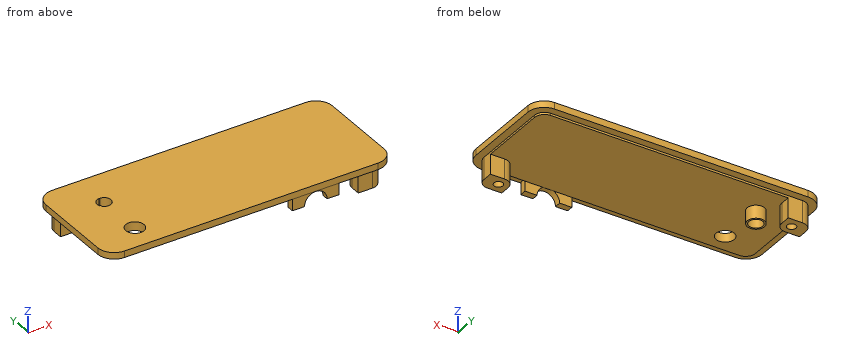
```python
from build123d import *

# Parameters (mm, degrees)
PAD002_DEPTH  = 1.5
PAD003_DEPTH  = 0.5
SKETCH005_R   = 1.025
PAD004_DEPTH  = 4.6
SKETCH006_R   = 2.1
POCKET_DEPTH  = 2
SKETCH008_R   = 2
SKETCH008_R_2 = 1.6
PAD005_DEPTH  = 3
PAD014_DEPTH  = 1.5


with BuildPart() as part:
    # Sketch003 → Pad002 (new body)
    with BuildSketch(Plane.XY.offset(6)):
        with BuildLine():
            Line((-29.25, 13), (29.25, 13))
            ThreePointArc((33, 9.25), (31.9016504294, 11.9016504294), (29.25, 13))
            Line((33, 9.25), (33, -9.25))
            ThreePointArc((29.25, -13), (31.9016504295, -11.9016504294), (33, -9.25))
            Line((29.25, -13), (-29.25, -13))
            ThreePointArc((-33, -9.25), (-31.9016504294, -11.9016504295), (-29.25, -13))
            Line((-33, -9.25), (-33, 9.25))
            ThreePointArc((-29.25, 13), (-31.9016504294, 11.9016504294), (-33, 9.25))
        make_face()
    extrude(amount=PAD002_DEPTH)

    # Sketch004 → Pad003 (new body)
    with BuildSketch(Plane(origin=(0, 0, 6), x_dir=(1, 0, 0), z_dir=(0, 0, -1))):
        with BuildLine():
            Line((-29.05, 11.3), (29.05, 11.3))
            ThreePointArc((31.3, 9.05), (30.6409902577, 10.6409902577), (29.05, 11.3))
            Line((31.3, 9.05), (31.3, -9.05))
            ThreePointArc((29.05, -11.3), (30.6409902577, -10.6409902577), (31.3, -9.05))
            Line((29.05, -11.3), (-29.05, -11.3))
            ThreePointArc((-31.3, -9.05), (-30.6409902577, -10.6409902577), (-29.05, -11.3))
            Line((-31.3, -9.05), (-31.3, 9.05))
            ThreePointArc((-29.05, 11.3), (-30.6409902577, 10.6409902577), (-31.3, 9.05))
        make_face()
    extrude(amount=PAD003_DEPTH)

    # Sketch005 → Pad004 (new body)
    with BuildSketch(Plane(origin=(0, 0, 5.5), x_dir=(1, 0, 0), z_dir=(0, 0, -1))):
        with BuildLine():
            Line((-25.75, -9), (-25.75, -11.3))
            Line((-25.75, -11.3), (-29.05, -11.3))
            ThreePointArc((-31.3, -9.05), (-30.6409902577, -10.6409902577), (-29.05, -11.3))
            Line((-31.3, -6.75), (-31.3, -9.05))
            Line((-27.9999999923, -6.75), (-31.3, -6.75))
            ThreePointArc((-25.75, -9.0000000077), (-26.4090097369, -7.4090097478), (-27.9999999923, -6.75))
        make_face()
        with Locations((-28, -9)):
            Circle(SKETCH005_R, mode=Mode.SUBTRACT)
        with BuildLine():
            ThreePointArc((25.75, 9), (26.4090097423, 7.4090097423), (28, 6.75))
            Line((28, 6.75), (31.3, 6.75))
            Line((31.3, 9.05), (31.3, 6.75))
            ThreePointArc((31.3, 9.05), (30.6409902577, 10.6409902577), (29.05, 11.3))
            Line((29.05, 11.3), (25.75, 11.3))
            Line((25.75, 11.3), (25.75, 9))
        make_face()
        with Locations((28, 9)):
            Circle(SKETCH005_R, mode=Mode.SUBTRACT)
    extrude(amount=PAD004_DEPTH)

    # Sketch006 → Pocket (cut)
    with BuildSketch(Plane.XY.offset(7.5)):
        with Locations((-23, -7)):
            Circle(SKETCH006_R)
        with BuildLine():
            ThreePointArc((-24.3288922086, 3.1089076939), (-23.0026761128, 2.400002238), (-21.6740960519, 3.1044673539))
            ThreePointArc((-21.5638430432, 3.2946963807), (-21.7108688116, 3.2528448762), (-21.6740960519, 3.1044673539))
            ThreePointArc((-21.5638430432, 3.2946963807), (-21.6130238799, 4.7976824194), (-22.8873953748, 5.5960326433))
            ThreePointArc((-23.1072650483, 5.5964003913), (-22.9975078699, 5.4899979159), (-22.8873953748, 5.5960326433))
            ThreePointArc((-23.1072650483, 5.5964003913), (-24.3843000035, 4.8023175806), (-24.4385082583, 3.2995044678))
            ThreePointArc((-24.3288922086, 3.1089076939), (-24.2916233116, 3.2571613762), (-24.4385082583, 3.2995044678))
        make_face()
    extrude(amount=-POCKET_DEPTH, mode=Mode.SUBTRACT)

    # Sketch008 → Pad005 (new body)
    with BuildSketch(Plane(origin=(0, 0, 5.5), x_dir=(1, 0, 0), z_dir=(0, 0, -1))):
        with Locations((-23, -4)):
            Circle(SKETCH008_R)
        with Locations((-23, -4)):
            Circle(SKETCH008_R_2, mode=Mode.SUBTRACT)
    extrude(amount=PAD005_DEPTH)

    # Sketch023 → Pad014 (new body)
    with BuildSketch(Plane(origin=(0, -11.3, 6), x_dir=(1, 0, 0), z_dir=(0, -1, 0))):
        with BuildLine():
            Line((9.6, 0), (20.4, 0))
            Line((20.4, 0), (20.4, -2.8))
            Line((20.4, -2.8), (17.6, -2.8))
            ThreePointArc((17.6, -2.8), (15, -0.2), (12.4, -2.8))
            Line((12.4, -2.8), (9.6, -2.8))
            Line((9.6, -2.8), (9.6, 0))
        make_face()
    extrude(amount=PAD014_DEPTH)


solid = part.part
```
Could you check a few things on this model? Use its own coordinates, in mm. Give positions to 0.01 mm unless a question says otherwise; leave off trailing zeros. Write each loop counter-clockwise with the first axis right and the second up, starting at its lowest first coordinate (ties: lowest second). Pieces come first, ordered by that corner, then holes. Notation, with made-up numbers: (1.25, 71.25) -> (30.25, 71.25) arc R18 ccw to (30.25, 106.25) -> close; hole circle Ø8 at (-23.75, 3). An arc over 180 degrees is marked (long way). Write each question's results on one line, items separated by ' | '.
1. I want a section at A-A, the plane z = 4. Write out the boundary of the cut face in (x, y) (3 decimals).
Check sheet entries:
outline: (-31.3, 6.75) -> (-28, 6.75) arc R2.25 ccw to (-25.75, 9) -> (-25.75, 11.3) -> (-29.05, 11.3) arc R2.25 ccw to (-31.3, 9.05) -> close; circle Ø4 at (-23, 4); (9.6, -12.8) -> (12.526, -12.8) -> (12.526, -11.3) -> (9.6, -11.3) -> close; (17.474, -12.8) -> (20.4, -12.8) -> (20.4, -11.3) -> (17.474, -11.3) -> close; (25.75, -11.3) -> (29.05, -11.3) arc R2.25 ccw to (31.3, -9.05) -> (31.3, -6.75) -> (28, -6.75) arc R2.25 ccw to (25.75, -9) -> close; hole circle Ø2.05 at (-28, 9); hole circle Ø3.2 at (-23, 4); hole circle Ø2.05 at (28, -9)
2. I want a section at D-D, the plane x = 15. Write out the boundary of the cut face in (y, z), then the cut area to 3 significant figures.
Check sheet entries:
outline: (-13, 6) -> (-12.8, 6) -> (-12.8, 5.8) -> (-11.3, 5.8) -> (-11.3, 5.5) -> (11.3, 5.5) -> (11.3, 6) -> (13, 6) -> (13, 7.5) -> (-13, 7.5) -> close | area: 50.6 mm²
3. I need wall thicknesses on L1, parallel to X at y = -9, z = 4.1 (3 decimals); L2, parallel to X at y = 3.25, z = 7.25; L3, parallel to Z at x = 28, y = -9. Which ranges of each line are inside material? Lowest first, please.
Check sheet entries:
L1: x = 25.75 to 26.975, 29.025 to 31.3 | L2: x = -33 to -24.29, -21.71 to 33 | L3: z = 5.5 to 7.5
4. Will these pins go through, and if not, where does the flat tip stop? pin 1 Ø1.8 at (y, z) = (-10.5, 3.5) entering from -X; pin 2 Ø0.7 at (x, z) = (17.5, 4.5) entering from +Y; pin 3 Ø1 at (x, y) = (-28, 9) entering from -Z.
Check sheet entries:
pin 1: stops at x = 9.6 | pin 2: stops at y = -11.3 | pin 3: stops at z = 5.5
5. I want a section at B-B, the plane x = -14. Write out the boundary of the cut face in (y, z), then the cut area to 3 significant figures.
Check sheet entries:
outline: (-13, 6) -> (-11.3, 6) -> (-11.3, 5.5) -> (11.3, 5.5) -> (11.3, 6) -> (13, 6) -> (13, 7.5) -> (-13, 7.5) -> close | area: 50.3 mm²
6. I want a section at C-C, the plane y = 1.25. Write out the boundary of the cut face in (x, z), then the cut area to 3 significant figures.
Check sheet entries:
outline: (-33, 6) -> (-31.3, 6) -> (-31.3, 5.5) -> (31.3, 5.5) -> (31.3, 6) -> (33, 6) -> (33, 7.5) -> (-33, 7.5) -> close | area: 130 mm²
